```python
from build123d import *

# Parameters (mm, degrees)
F0_R     = 76.2
F1_DEPTH = 635
F3_D     = 101.6
F4_SIZE  = 6.35
F5_SIZE  = 6.35


with BuildPart() as f1:
    # F0 (on Front) → F1 (new body)
    with BuildSketch(Plane.XZ):
        Circle(F0_R)
    extrude(amount=F1_DEPTH)

    # F3 (through all)
    with Locations(Plane.XZ.offset(635)):
        with Locations((0, 0)):
            Hole(F3_D / 2)

    # F4
    f4_edges = [f1.edges().sort_by_distance(p)[0] for p in [
        (-76.2, -635, 0),
    ]]
    chamfer(f4_edges, length=F4_SIZE)

    # F5
    f5_edges = [f1.edges().sort_by_distance(p)[0] for p in [
        (-76.2, 0, 0),
    ]]
    chamfer(f5_edges, length=F5_SIZE)


solid = f1.part
```
Verification items for the finished model (mm, model axes). Coordinates: 2 decimals unless noted, no trailing zeros. Order: outer loops, then holes, each group sorted by start corner. A loop starts at its lowest first (then second) coordinate and runs counter-clockwise, first axis right, second up. Notation, with made-up numbers: (-40, -4) - (9, -4) arc R32 cw to (9, 25) - close; hole circle Ø8 at (22.5, -11). An arc over 180 degrees is marked (long way). Return JSON: item names as keys, results as strings.
(1) Section check B-B, the plane z = 0. Record the cut outline in (x, y), and give its area (3 significant figures).
Filled sheet:
{"outline": "(-76.2, -628.65) - (-69.85, -635) - (-50.8, -635) - (-50.8, 0) - (-69.85, 0) - (-76.2, -6.35) - close; (50.8, -635) - (69.85, -635) - (76.2, -628.65) - (76.2, -6.35) - (69.85, 0) - (50.8, 0) - close", "area": "32,200 mm^2"}
(2) Section check A-A, the plane x = 0. Record the cut outline in (y, z), and give its area (3 significant figures).
Filled sheet:
{"outline": "(-635, -69.85) - (-628.65, -76.2) - (-6.35, -76.2) - (0, -69.85) - (0, -50.8) - (-635, -50.8) - close; (-635, 50.8) - (0, 50.8) - (0, 69.85) - (-6.35, 76.2) - (-628.65, 76.2) - (-635, 69.85) - close", "area": "32,200 mm^2"}
(3) Thickness scan on line 1 along X through (y, z) = (-191.5, -0.5); line 2 along Z through (x, y) = (20, -468). Record the ranges inside material, lowest first.
Filled sheet:
{"line 1": "x = -76.2 to -50.8, 50.8 to 76.2", "line 2": "z = -73.53 to -46.7, 46.7 to 73.53"}
(4) Go/stop test with flat-tipped pins: pin 1 (12 mm diameter, centred on x = -46.5, y = -373.5, fed in from -Z); pin 2 (4 mm diameter, centred on x = -10, y = -259, fed in from -Z); pin 3 (2 mm diameter, centred on y = -363, z = -21, fed in from +X). Record where each tip stops, or that it passes through.
Filled sheet:
{"pin 1": "stops at z = -64.55", "pin 2": "stops at z = -75.78", "pin 3": "stops at x = 73.53"}
(5) Mould release check, pull along Z, two halves, no side actions. Record for faces 1 (the flat face through (5, -635, -51)), 2 (the conical face through (-55.68, -0.31, -42.69)), 3 (the cylindrical face through (11.012, -313.055, -49.592)): pulls with the +Z half, pulls with the -Z half, needs draft (parallel to the pull), parting line crosses it, or undercut.
Filled sheet:
{"face 1": "needs draft", "face 2": "parting line crosses it", "face 3": "undercut"}
(6) Section check C-C, the plane y = -344.5. Record the cut outline in (x, z), and give its area (3 significant figures).
Filled sheet:
{"outline": "circle Ø152.4 at (0, 0); hole circle Ø101.6 at (0, 0)", "area": "10,100 mm^2"}
